The drawing under review shows one solid part. Ordinate dimensions are in mm from its lowest x, y, z. A direction names the side the tool comes from. Give positions to 0.01 mm unless a question says otherwise; leave off trailing zeros. Write each loop counter-clockwise with the first axis right and the second up, starting at its lowest first coordinate (ties: lowest second). Pieces come first, ordered by that corner, then holes. Notation, with made-up numbers: M -24.5,25.25 L 24.5,25.25 A16 cw 24.5,50.25 Z; hole C 46.5,55 d2. An arc over 180 degrees is marked long. Write each question's results on one line, items separated by ' | '. Start each with the question number.
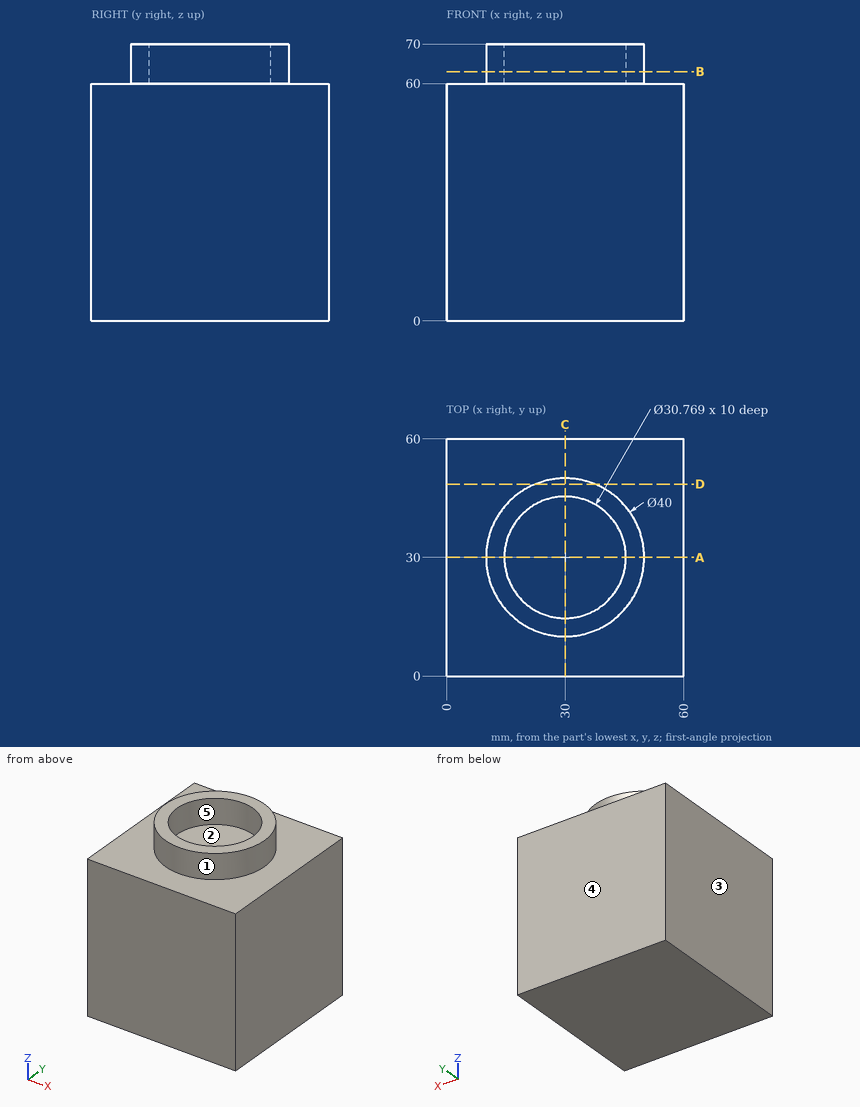
Q1. For pin 1 Ø18.5 at (x, y) = (30, 30) entering from +Z, flat-tipped, find the tip position at first contact; note if it passes through.
Q2. We need section A-A on y = 30. Write out the cut boundary in (x, z), and give its area (3 significant figures).
Q3. We need section D-D on y = 48.5. Write out the cut boundary in (x, z).
Q4. Wall thickness on line 1 along Y through (x, z) = (30, 67.25); line 2 along Z through (x, y) = (13, 44); line 3 along X through (y, z) = (27, 63): over which ranges is each line inside the solid? List them lowest first. Write a range as from..to.
Q5. The part is to be moulded in two halves that separate along X. For the marked faces 1, 2 and 3, say which applies: pulls with the +X half, pulls with the -X half, needs draft (parallel to the pull), parting line crosses it, or undercut.
Q6. We need section B-B on z = 63. Write out the cut boundary in (x, y).
Q7. For the marked faces 4 and 5, list the 3-axis set-ups (+Z, -Z, +X, -X, +Y, -Y) from which the entire face can be reached by the end or side of a thin tool; tool diameter is ignored.
Answer sheet:
1) pin 1: z = 60
2) outline: M 0,0 L 60,0 L 60,60 L 50,60 L 50,70 L 45.38,70 L 45.38,60 L 14.62,60 L 14.62,70 L 10,70 L 10,60 L 0,60 Z | area: 3,690 mm^2
3) outline: M 0,0 L 60,0 L 60,60 L 37.6,60 L 37.6,70 L 22.4,70 L 22.4,60 L 0,60 Z
4) line 1: 10..14.62, 45.38..50 | line 2: 0..60 | line 3: 10.23..14.91, 45.09..49.77
5) face 1: parting line crosses it | face 2: undercut | face 3: pulls with the -X half
6) outline: C 30,30 d40; hole C 30,30 d30.77
7) face 4: +Z, -Z, +X, -X, +Y | face 5: +Z
